For this review, take the finished solid that the model builds, in its own axes (mm). Give positions to 0.01 mm unless a question says otherwise; leave off trailing zeros. Order: outer loops, then holes, each group sorted by start corner. A loop starts at its lowest first (then second) coordinate and runs counter-clockwise, first axis right, second up. Notation, with made-up numbers: (-27, 75.25) - (23, 75.25) arc R30 cw to (23, 113.25) - close; hole circle Ø8 at (50, 72). An arc over 180 degrees is marked (long way). Answer as a JSON object with one key per item and string values. Group by question number.
from build123d import *

# Parameters (mm, degrees)
SKETCH1_W          = 200.025
SKETCH1_H          = 212.725
EXTRUDE1_DEPTH     = 6.35
CUT_EXTRUDE1_REACH = 152.553
SKETCH2_W          = 149.225
SKETCH2_H          = 9.525


with BuildPart() as part:
    # Sketch1 → Extrude1 (new body)
    with BuildSketch(Plane.XY):
        with Locations((6.35, 0)):
            Rectangle(SKETCH1_W, SKETCH1_H)
    extrude(amount=EXTRUDE1_DEPTH)

    # Sketch2 → Cut-Extrude1 (cut, up to next)
    with BuildSketch(Plane.XY.offset(6.35), mode=Mode.PRIVATE) as cut_extrude1_sk1:
        with Locations((6.35, -101.6)):
            Rectangle(SKETCH2_W, SKETCH2_H)
    cut_extrude1_tool1 = extrude(cut_extrude1_sk1.sketch, amount=-CUT_EXTRUDE1_REACH, mode=Mode.PRIVATE) & part.part
    cut_extrude1 = cut_extrude1_tool1.solids().sort_by_distance((6.35, -101.6, 6.35))[0]
    add(cut_extrude1, mode=Mode.SUBTRACT)

    # Mirror1: Cut-Extrude1 across plane
    add(cut_extrude1.mirror(Plane.ZX), mode=Mode.SUBTRACT)


solid = part.part
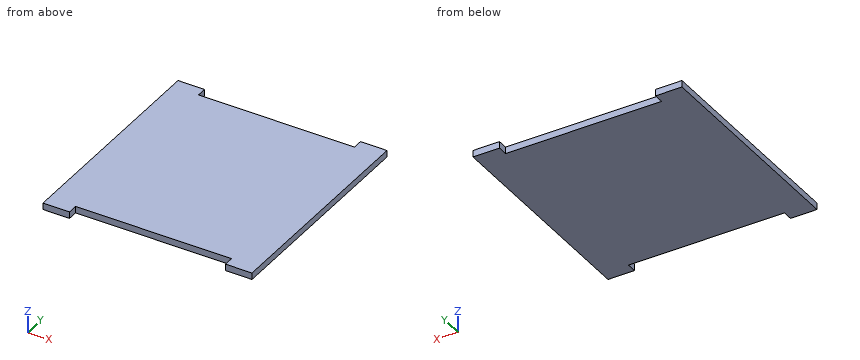
1) Consider section B-B (x = -56.5). Give the boundary of the cut face in (y, z), plus the area to 3 significant figures.
2) For line 1 (Y direction, x = 71, z = 0.75), list the stretches that pass through material, from the lowest coordinate up.
3) Consider section A-A (z = 2.5). Give the boundary of the cut face in (x, y), plus the area to 3 significant figures.
4) For pin 1 (3 mm diameter, centred on x = 45.5, z = 3.5, fed in from -Y); pin 2 (1.9 mm diameter, centred on x = 36.5, z = 4.5, fed in from +Y), all flat-tipped, find the tip position at first contact; note any pin that passes through.
Result set:
{
 "1": {"outline": "(-96.84, 0) - (96.84, 0) - (96.84, 6.35) - (-96.84, 6.35) - close", "area": "1,230 mm2"},
 "2": {"line 1": "y = -96.84 to 96.84"},
 "3": {"outline": "(-93.66, -106.36) - (-68.26, -106.36) - (-68.26, -96.84) - (80.96, -96.84) - (80.96, -106.36) - (106.36, -106.36) - (106.36, 106.36) - (80.96, 106.36) - (80.96, 96.84) - (-68.26, 96.84) - (-68.26, 106.36) - (-93.66, 106.36) - close", "area": "39,700 mm2"},
 "4": {"pin 1": "stops at y = -96.84", "pin 2": "stops at y = 96.84"}
}
